```python
from build123d import *

# Parameters (mm, degrees)
SKETCH_W        = 46.5
SKETCH_H        = 54.5
PAD_DEPTH       = 67
THICKNESS_T     = 1
SKETCH001_W     = 6
SKETCH001_H     = 6
PAD001_DEPTH    = 12
CHAMFER_SIZE    = 5.9
SKETCH002_R     = 1.25
POCKET_DEPTH    = 6
SKETCH003_W     = 17.5
SKETCH003_H     = 68
POCKET001_DEPTH = 1
POCKET002_DEPTH = 1


with BuildPart() as part:
    # Sketch → Pad (new body)
    with BuildSketch(Plane.XY):
        with Locations((0, -5.25)):
            Rectangle(SKETCH_W, SKETCH_H)
    extrude(amount=PAD_DEPTH)

    # Thickness
    thickness_openings = [part.faces().sort_by_distance(p)[0] for p in [
        (0, -5.25, 67),
    ]]
    offset(amount=THICKNESS_T, openings=thickness_openings)

    # Sketch001 → Pad001 (new body)
    with BuildSketch(Plane.XY.offset(67)):
        with Locations((-27.25, 18)):
            Rectangle(SKETCH001_W, SKETCH001_H)
        with Locations((27.25, -18)):
            Rectangle(SKETCH001_W, SKETCH001_H)
    extrude(amount=-PAD001_DEPTH)

    # Chamfer
    chamfer_edges = [part.edges().sort_by_distance(p)[0] for p in [
        (-30.25, 18, 55),
        (30.25, -18, 55),
    ]]
    chamfer(chamfer_edges, length=CHAMFER_SIZE)

    # Sketch002 → Pocket (cut)
    with BuildSketch(Plane.XY.offset(67)):
        with Locations((-27.25, 18)):
            Circle(SKETCH002_R)
        with Locations((27.25, -18)):
            Circle(SKETCH002_R)
    extrude(amount=-POCKET_DEPTH, mode=Mode.SUBTRACT)

    # Sketch003 → Pocket001 (cut)
    with BuildSketch(Plane.XZ.offset(33.5)):
        with Locations((0, 33)):
            Rectangle(SKETCH003_W, SKETCH003_H)
    extrude(amount=-POCKET001_DEPTH, mode=Mode.SUBTRACT)

    # Sketch004 → Pocket002 (cut)
    with BuildSketch(Plane(origin=(0, 0, -1), x_dir=(1, 0, 0), z_dir=(0, 0, -1))):
        with BuildLine():
            ThreePointArc((-3, 29), (0, 26), (3, 29))
            Line((3, 29), (3, 39))
            ThreePointArc((3, 39), (0, 42), (-3, 39))
            Line((-3, 29), (-3, 39))
        make_face()
    extrude(amount=-POCKET002_DEPTH, mode=Mode.SUBTRACT)


solid = part.part
```
Geometry: final body of the model. Coordinates: model frame, mm. A direction names the side the tool comes from. Give positions to 0.01 mm unless a question says otherwise; leave off trailing zeros. Order: outer loops, then holes, each group sorted by start corner. A loop starts at its lowest first (then second) coordinate and runs counter-clockwise, first axis right, second up. Notation, with made-up numbers: (-7, -1) -> (44, -1) arc R20 ccw to (44, 18) -> close; hole circle Ø9 at (38.5, 53.25). An arc over 180 degrees is marked (long way). Write each question's results on one line, items separated by ' | '. Start each with the question number.
1) First-contact query: pin 1 (4 mm diameter, centred on y = -12.5, z = 7.5, fed in from -X); pin 2 (5 mm diameter, centred on x = -26.5, z = 59.5, fed in from -Y); pin 3 (5 mm diameter, centred on x = -16.5, y = -11.5, fed in from +Z); pin 4 (3 mm diameter, centred on x = 27.25, y = -18, fed in from +Z). Flat tips, straight axial feed; report the tip coordinate or a pass-through.
2) Draft query along Y for faces 1 (the flat face through (24.25, -6, 33)), 2 (the flat face through (0, 23, 33)), 3 (the flat face through (23.25, -6, 33)). Return one class per face: pulls with the +Y half, pulls with the -Y half, needs draft (parallel to the pull), parting line crosses it, or undercut.
3) Section C-C (z = 21.5). Return loops of the section in (x, y), then the cut area to 3 significant figures.
4) Section B-B (x = -17). Return loops of the section in (y, z).
5) Line query: line 1 (Y direction, x = -18.5, z = 8); line 2 (Y direction, x = 27.25, z = 64.85); line 3 (X direction, y = 2, z = 24.5). Output: solid intervals per line, ascending. Write a range as from..to.
6) Section A-A (y = 5). Return loops of the section in (x, z), then the cut area to 3 significant figures.
7) Section D-D (x = -27.25). Return loops of the section in (y, z), then the cut area to 3 significant figures.
8) Set-up query: faces 4 (the flat face through (0, -5, 0)), 5 (the flat face through (0, -5, -1)), 6 (the flat face through (-27, 21, 62)), 7 (the flat face through (27, -21, 62)). Return all of +Z, -Z, +X, -X, +Y, -Y with unobstructed straight access to the full face (end or side cutting, diameter ignored); none if empty.
Calculated:
1) pin 1: x = -24.25 | pin 2: y = -33.16 | pin 3: z = 0 | pin 4: z = 67
2) face 1: needs draft | face 2: pulls with the +Y half | face 3: undercut
3) outline: (-24.25, -32.5) arc R1 ccw to (-23.25, -33.5) -> (-8.75, -33.5) -> (-8.75, -32.5) -> (-23.25, -32.5) -> (-23.25, 22) -> (23.25, 22) -> (23.25, -32.5) -> (8.75, -32.5) -> (8.75, -33.5) -> (23.25, -33.5) arc R1 ccw to (24.25, -32.5) -> (24.25, 22) arc R1 ccw to (23.25, 23) -> (-23.25, 23) arc R1 ccw to (-24.25, 22) -> close | area: 188 mm2
4) outline: (-33.5, 0) arc R1 ccw to (-32.5, -1) -> (22, -1) arc R1 ccw to (23, 0) -> (23, 67) -> (22, 67) -> (22, 0) -> (-32.5, 0) -> (-32.5, 67) -> (-33.5, 67) -> close
5) line 1: -33.5..-32.5, 22..23 | line 2: -21..-19.25, -16.75..-15 | line 3: -24.25..-23.25, 23.25..24.25
6) outline: (-24.25, 0) arc R1 ccw to (-23.25, -1) -> (23.25, -1) arc R1 ccw to (24.25, 0) -> (24.25, 67) -> (23.25, 67) -> (23.25, 0) -> (-23.25, 0) -> (-23.25, 67) -> (-24.25, 67) -> close | area: 182 mm2
7) outline: (15, 57.9) -> (21, 57.9) -> (21, 67) -> (19.25, 67) -> (19.25, 61) -> (16.75, 61) -> (16.75, 67) -> (15, 67) -> close | area: 39.6 mm2
8) face 4: +Z | face 5: -Z, +X, -X, +Y, -Y | face 6: +Z, -Z, -X, +Y | face 7: +Z, -Z, +X, -Y
